```python
from build123d import *

# Parameters (mm, degrees)
SKETCH1_W           = 100
SKETCH1_H           = 70
BOSS_EXTRUDE1_DEPTH = 10
SKETCH2_W           = 70
SKETCH2_H           = 10
BOSS_EXTRUDE3_DEPTH = 100
SKETCH3_R           = 7.5
BOSS_EXTRUDE4_DEPTH = 30
SKETCH4_R           = 7.65
BOSS_EXTRUDE5_DEPTH = 30
SKETCH5_R           = 7.65
BOSS_EXTRUDE6_DEPTH = 30


with BuildPart() as part:
    # Sketch1 → Boss-Extrude1 (new body)
    with BuildSketch(Plane.XY):
        Rectangle(SKETCH1_W, SKETCH1_H)
    extrude(amount=BOSS_EXTRUDE1_DEPTH)

    # Sketch2 → Boss-Extrude3 (add)
    with BuildSketch(Plane.ZY.offset(50)):
        with Locations((45, -30)):
            Rectangle(SKETCH2_W, SKETCH2_H)
    extrude(amount=-BOSS_EXTRUDE3_DEPTH)

    # Sketch3 → Boss-Extrude4 (add)
    with BuildSketch(Plane(origin=(0, 0, 0), x_dir=(-1, 0, 0), z_dir=(0, 0, -1))):
        with Locations(Location((0, 15, 0), (0, 0, 180))):
            Circle(SKETCH3_R)
    extrude(amount=BOSS_EXTRUDE4_DEPTH)

    # Sketch4 → Boss-Extrude5 (add)
    with BuildSketch(Plane(origin=(0, 0, 0), x_dir=(-1, 0, 0), z_dir=(0, 0, -1))):
        with Locations((0, 15.3)):
            Circle(SKETCH4_R)
    extrude(amount=BOSS_EXTRUDE5_DEPTH)

    # Sketch5 → Boss-Extrude6 (add)
    with BuildSketch(Plane(origin=(0, 0, 0), x_dir=(-1, 0, 0), z_dir=(0, 0, -1))):
        with Locations((0.3, 15)):
            Circle(SKETCH5_R)
    extrude(amount=BOSS_EXTRUDE6_DEPTH)


solid = part.part
```
Could you check a few things on this model? Use its own coordinates, in mm. A direction names the side the tool comes from. Round coordinates to 2 decimals unless told otherwise and drop trailing zeros. Write each loop counter-clockwise with the first axis right and the second up, starting at its lowest first coordinate (ties: lowest second). Pieces come first, ordered by that corner, then holes. Notation, with made-up numbers: M 22.25,-4.75 L 63.25,-4.75 A24 cw 63.25,19.25 Z; hole C 24,-1.5 d1. An arc over 180 degrees is marked long. Write each question's results on one line, items separated by ' | '. Start each with the question number.
1. I need wall thicknesses on L1, parallel to Z at x = 36.5, y = -1.5; L2, parallel to Z at x = 32, y = -26; L3, parallel to Y at x = 22.5, z = 51. Which ranges of each line are inside material? Lowest first, please. Write a range as from..to.
2. I'm going to push flat-ended pins straight in: pin 1 Ø8 at (x, y) = (24, -21.5) entering from -Z; pin 2 Ø6 at (x, y) = (24, -20) entering from +Z. Where does each tip first touch, or does it pass through?
3. Imagine slicing it at A-A on y = -21. List the corners of the cut face in (x, z) for me.
4. Imagine slicing it at B-B on z = 28. List the corners of the cut face in (x, y) for me, and give its area (3 significant figures).
5. On a 3-axis mill with a long thin cutter (end or side, diameter ignored), from which of +Z, -Z, +X, -X, +Y, -Y can I reach the whole of each face in a straight line? I mean faces 1 (the face through (-1, -30, 80)), 2 (the face through (4.499, 21.487, -14.79)), 3 (the face through (5.324, 9.717, -14.79)), 4 (the face through (-1, 5, 10)). Say none if no direction works.
6. Imagine slicing it at C-C on x = 15.5. List the corners of the cut face in (y, z) for me.
7. Imagine slicing it at D-D on z = -2. List the corners of the cut face in (x, y) for me.
Result sheet:
1) L1: z = 0..10 | L2: z = 0..80 | L3: y = -35..-25
2) pin 1: stops at z = 0 | pin 2: stops at z = 10
3) outline: M -50,0 L 50,0 L 50,10 L -50,10 Z
4) outline: M -50,-35 L 50,-35 L 50,-25 L -50,-25 Z | area: 1,000 mm^2
5) face 1: +Z, +X, -X, +Y, -Y | face 2: -Z | face 3: -Z, +X, -Y | face 4: +Z, +X, -X, +Y
6) outline: M -35,0 L 35,0 L 35,10 L -25,10 L -25,80 L -35,80 Z
7) outline: M -5.56,20.56 A7.65 ccw 3.64,8.44 A7.5 ccw 6.56,11.36 A7.65 ccw Z
